Source: CAD feature listing. Evaluate the final solid. Frame: model axes, mm. A direction names the side the tool comes from. Give positions to 0.01 mm unless a question says otherwise; leave off trailing zeros. Order: outer loops, then holes, each group sorted by start corner. A loop starts at its lowest first (then second) coordinate and runs counter-clockwise, first axis right, second up.
```python
from build123d import *

# Parameters (mm, degrees)
F1_DEPTH = 10.16
F3_DEPTH = 6.35
F5_DEPTH = 10.161
F7_D     = 2.7051
F7_DEPTH = 4.76885
F7_TIP   = 0.8126940303


with BuildPart() as f1:
    # F0 (on Top) → F1 (new body)
    with BuildSketch(Plane.XY):
        with BuildLine():
            Line((25.4, 7.62), (7.62, 7.62))
            ThreePointArc((7.62, 7.62), (0, 0), (7.62, -7.62))
            Line((7.62, -7.62), (25.4, -7.62))
            Line((25.4, -7.62), (32.023525542, -18.016852513))
            ThreePointArc((32.023525542, -18.016852513), (34.3247825403, -20.1722148987), (37.3790612229, -20.955))
            Line((37.3790612229, -20.955), (44.45, -20.955))
            Line((44.45, -20.955), (44.45, 20.955))
            Line((44.45, 20.955), (37.3790612229, 20.955))
            ThreePointArc((37.3790612229, 20.955), (34.3247825403, 20.1722148987), (32.023525542, 18.016852513))
            Line((32.023525542, 18.016852513), (25.4, 7.62))
        make_face()
    extrude(amount=F1_DEPTH)

    # F2 (on face) → F3 (cut)
    with BuildSketch(Plane.XY.offset(10.16)):
        with BuildLine():
            ThreePointArc((7.62, 5.08), (2.54, 0), (7.62, -5.08))
            Line((7.62, -5.08), (17.78, -5.08))
            ThreePointArc((17.78, -5.08), (22.86, 0), (17.78, 5.08))
            Line((17.78, 5.08), (7.62, 5.08))
        make_face()
    extrude(amount=-F3_DEPTH, mode=Mode.SUBTRACT)

    # F4 (on Top) → F5 (cut, through all)
    with BuildSketch(Plane.XY):
        with BuildLine():
            ThreePointArc((7.62, 3.81), (3.81, 0), (7.62, -3.81))
            Line((7.62, -3.81), (17.78, -3.81))
            ThreePointArc((17.78, -3.81), (21.59, 0), (17.78, 3.81))
            Line((17.78, 3.81), (7.62, 3.81))
        make_face()
    extrude(amount=F5_DEPTH, mode=Mode.SUBTRACT)

    # F7
    with Locations(Plane.XY.offset(10.16)):
        with Locations((29.845, 0)):
            Hole(F7_D / 2, depth=F7_DEPTH)
            with Locations((0, 0, -(F7_DEPTH + F7_TIP / 2))):  # 118° drill point
                Cone(0, F7_D / 2, F7_TIP, mode=Mode.SUBTRACT)


solid = f1.part
```
1) Pin query (flat end, axial travel): pin 1 (10 mm diameter, centred on x = 18, y = 2.5, fed in from -Z); pin 2 (5 mm diameter, centred on x = 17.5, z = 7.5, fed in from -Y); pin 3 (5 mm diameter, centred on y = 16.5, z = 1, fed in from -X); pin 4 (4 mm diameter, centred on x = 11, z = 1.5, fed in from +Y). Return the tip coordinate at first contact, or that it passes through.
Report:
pin 1: stops at z = 0
pin 2: stops at y = -7.62
pin 3: stops at x = 29.46
pin 4: stops at y = 7.62
2) Material intervals for L1, parallel to X at y = 0, z = 8.2; L2, parallel to Y at x = 12.5, z = 5.25; L3, parallel to Y at x = 10, z = 0.75, sorted ascending.
Report:
L1: x = 0 to 2.54, 22.86 to 28.49, 31.2 to 44.45
L2: y = -7.62 to -5.08, 5.08 to 7.62
L3: y = -7.62 to -3.81, 3.81 to 7.62
3) Reachability of faces 1 (the cylindrical face through (2.54, 0.11, 7.03)), 2 (the flat face through (13, 3.81, 2)), 3 (the flat face through (17, 7.62, 5)) from +Z, -Z, +X, -X, +Y, -Y: full face, straight path, thin tool, end or side. Return the list, or none.
Report:
face 1: +Z
face 2: +Z, -Z
face 3: +Z, -Z, -X, +Y
4) Section query A-A, the plane z = 7.5. Return the cut outline in (x, y) (3 decimals), and give its area (3 significant figures).
Report:
outline: (7.62, -7.62) - (25.4, -7.62) - (32.024, -18.017) arc R6.35 ccw to (37.379, -20.955) - (44.45, -20.955) - (44.45, 20.955) - (37.379, 20.955) arc R6.35 ccw to (32.024, 18.017) - (25.4, 7.62) - (7.62, 7.62) arc R7.62 ccw to start; hole (7.62, -5.08) - (17.78, -5.08) arc R5.08 ccw to (17.78, 5.08) - (7.62, 5.08) arc R5.08 ccw to start; hole circle Ø2.705 at (29.845, 0)
area: 853 mm2
5) Section query D-D, the plane y = 16. Return the cut outline in (x, z), and give its area (3 significant figures).
Report:
outline: (30.74, 0) - (44.45, 0) - (44.45, 10.16) - (30.74, 10.16) - close
area: 139 mm2
6) Section query B-B, the plane x = 5. Return the cut outline in (y, z), and give its area (3 significant figures).
Report:
outline: (-7.16, 0) - (-2.77, 0) - (-2.77, 3.81) - (-4.35, 3.81) - (-4.35, 10.16) - (-7.16, 10.16) - close; (2.77, 0) - (7.16, 0) - (7.16, 10.16) - (4.35, 10.16) - (4.35, 3.81) - (2.77, 3.81) - close
area: 69.0 mm2
7) Section query C-C, the plane y = 2. Return the cut outline in (x, z).
Report:
outline: (0.27, 0) - (4.38, 0) - (4.38, 3.81) - (2.95, 3.81) - (2.95, 10.16) - (0.27, 10.16) - close; (21.02, 0) - (44.45, 0) - (44.45, 10.16) - (22.45, 10.16) - (22.45, 3.81) - (21.02, 3.81) - close
8) Draft query along Y for faces 4 (the flat face through (16, -7.62, 5)), 5 (the flat face through (13, -5.08, 7)), 6 (the cylindrical face through (34.36, 20.19, 5.01)), 7 (the flat face through (13, -3.81, 2)). Return one class per face: +Y half, -Y half, draft (parallel to the pull), parting line (faces both ways), or undercut.
Report:
face 4: -Y half
face 5: undercut
face 6: +Y half
face 7: undercut
